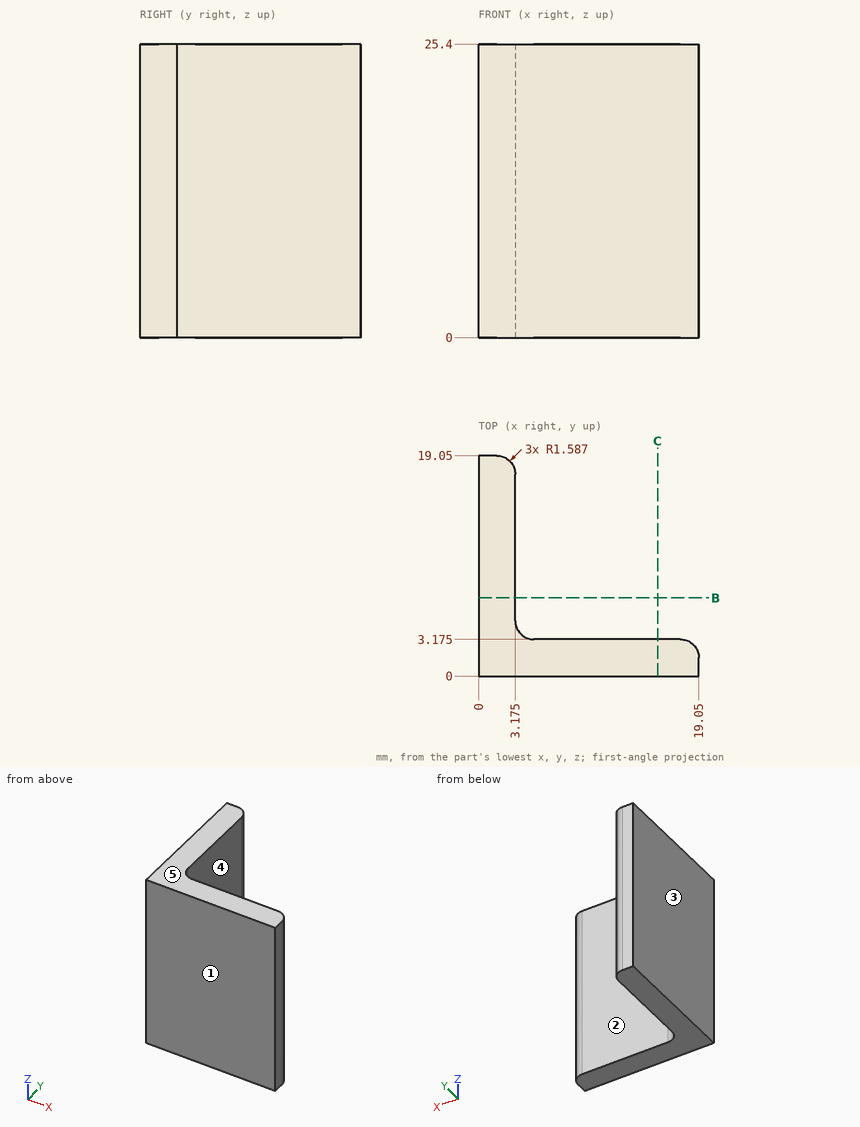
Geometry check sheet. Reference: drawing and pictorial views, mm from the part's lowest x, y, z. A direction names the side the tool comes from. Give positions to 0.01 mm unless a question says otherwise; leave off trailing zeros. Order: outer loops, then holes, each group sorted by start corner. A loop starts at its lowest first (then second) coordinate and runs counter-clockwise, first axis right, second up. Notation, with made-up numbers: M 8,85 L 56,85 A29 ccw 56,117 Z; hole C 13,-9.5 d9. An arc over 180 degrees is marked long. Answer in a Markdown table with one row per item.
1) Gauge pin test, flat ends, axial feed: P1, Ø1.5, axis at x = 10.5, z = 12.5, coming from the +Y side (1 decimal); P2, Ø10, axis at x = 9, z = 7, coming from the +Y side; P3, Ø6.5, axis at y = 14, z = 13.5, coming from the +X side (1 decimal). Record the tip position at first contact, or that the pin passes through.
Filled sheet:
| item | result |
|---|---|
| P1 | stops at y = 3.2 |
| P2 | stops at y = 3.37 |
| P3 | stops at x = 3.2 |
2) Cross-section at B-B, the plane y = 6.75. Enter the section's corners in (x, z) (1 decimal).
Filled sheet:
| item | result |
|---|---|
| outline | M 0,0 L 3.2,0 L 3.2,25.4 L 0,25.4 Z |
3) Release check for a two-part mould opening along X. For the marked faces 3, 4 and 5 record: +X half, -X half, draft (parallel to the pull), parting line (faces both ways), or undercut.
Filled sheet:
| item | result |
|---|---|
| face 3 | -X half |
| face 4 | +X half |
| face 5 | draft |
4) Thickness scan on L1, parallel to X at y = 13.5, z = 23.75 (1 decimal); L2, parallel to X at y = 18.25, z = 9 (1 decimal). Record the ranges inside material, lowest first. Write a range as [from, to].
Filled sheet:
| item | result |
|---|---|
| L1 | x = [0, 3.2] |
| L2 | x = [0, 3] |
5) Access from +Z, -Z, +X, -X, +Y, -Y to the whole of each face (thin tool, end or side, straight path). Record for the marked faces 1 and 2.
Filled sheet:
| item | result |
|---|---|
| face 1 | +Z, -Z, +X, -X, -Y |
| face 2 | +Z, -Z, +X, +Y |
